```python
from build123d import *

# Parameters (mm, degrees)
F1_DEPTH = 20.6375
F2_W     = 9.525
F2_H     = 28.575
F3_DEPTH = 47.625
F4_W     = 9.525
F4_H     = 28.575
F5_DEPTH = 47.625
F6_W     = 1104.9
F6_H     = 7.9375
F7_DEPTH = 9.525


with BuildPart() as f1:
    # F0 (on Front) → F1 (new body)
    with BuildSketch(Plane.XZ):
        with BuildLine():
            Line((552.45, 0), (0, 0))
            Line((0, 0), (-552.45, 0))
            Line((-552.45, 0), (-552.45, -88.9))
            ThreePointArc((-552.45, -88.9), (0, -69.85), (552.45, -88.9))
            Line((552.45, -88.9), (552.45, 0))
        make_face()
    extrude(amount=-F1_DEPTH)

    # F2 (on face) → F3 (join)
    with BuildSketch(Plane(origin=(-552.45, 0, 0), x_dir=(0, -1, 0), z_dir=(-1, 0, 0))):
        with Locations((-10.31875, -23.8125)):
            Rectangle(F2_W, F2_H)
        with Locations((-10.31875, -65.0875)):
            Rectangle(F2_W, F2_H)
    extrude(amount=F3_DEPTH)

    # F4 (on face) → F5 (join)
    with BuildSketch(Plane.YZ.offset(552.45)):
        with Locations((10.31875, -23.8125)):
            Rectangle(F4_W, F4_H)
        with Locations((10.31875, -65.0875)):
            Rectangle(F4_W, F4_H)
    extrude(amount=F5_DEPTH)

    # F6 (on face) → F7 (cut)
    with BuildSketch(Plane.XY):
        with Locations((0, 10.31875)):
            Rectangle(F6_W, F6_H)
    extrude(amount=-F7_DEPTH, mode=Mode.SUBTRACT)


solid = f1.part
```
Here's how the part is built. I have some questions about the finished solid (model axes, mm). A direction names the side the tool comes from. Coordinates: 2 decimals unless noted, no trailing zeros. Order: outer loops, then holes, each group sorted by start corner. A loop starts at its lowest first (then second) coordinate and runs counter-clockwise, first axis right, second up. Notation, with made-up numbers: (36.5, 73.25) -> (61.5, 73.25) arc R31 cw to (61.5, 100.25) -> close; hole circle Ø5 at (61.25, 64.5). An arc over 180 degrees is marked (long way). Return JSON: item names as keys, results as strings.
1) I'm going to push flat-ended pins straight in: P1, Ø6, axis at y = 13.5, z = -46.5, coming from the +X side; P2, Ø5, axis at x = -576.5, y = 8, coming from the -Z side (3 decimals); P3, Ø23, axis at x = -587, z = -20.5, coming from the +Y side. Where does each tip first touch, or does it pass through?
Conclusion:
{"P1": "stops at x = 552.45", "P2": "stops at z = -79.375", "P3": "stops at y = 15.08"}
2) If we section it at A-A on y = 11: List the corners of the cut face in (x, z) for me (3 decimals), plus the area to 3 significant figures.
Conclusion:
{"outline": "(-600.075, -79.375) -> (-552.45, -79.375) -> (-552.45, -88.9) arc R8020.05 cw to (552.45, -88.9) -> (552.45, -79.375) -> (600.075, -79.375) -> (600.075, -50.8) -> (552.45, -50.8) -> (552.45, -38.1) -> (600.075, -38.1) -> (600.075, -9.525) -> (-600.075, -9.525) -> (-600.075, -38.1) -> (-552.45, -38.1) -> (-552.45, -50.8) -> (-600.075, -50.8) -> close", "area": "79,100 mm²"}
3) If I drill on probe 1 along X at (y, z) = (18.25, -30.5); probe 2 along Z at (x, y) = (-311.5, 5.75); probe 3 along Z at (x, y) = (-497, 8.5) (3 decimals), over which ranges is the centre line in solid material (lowest first)?
Conclusion:
{"probe 1": "x = -552.45 to 552.45", "probe 2": "z = -75.9 to 0", "probe 3": "z = -85.264 to -9.525"}
4) On a 3-axis mill with a long thin cutter (end or side, diameter ignored), from which of +Z, -Z, +X, -X, +Y, -Y can I reach the whole of each face in a straight line? I mean faces 1 (the flat face through (-576, 15.081, -65)), 2 (the flat face through (576, 15.081, -24)), 3 (the flat face through (576, 5.556, -65)). Say none if no direction works.
Conclusion:
{"face 1": "+Z, -Z, -X, +Y", "face 2": "+Z, -Z, +X, +Y", "face 3": "+Z, -Z, +X, -Y"}
5) Thinking about a two-plate mould opening in X: for faces 4 (the flat face through (576, 15.081, -65)), 5 (the cylindrical face through (-7.74, 10.174, -69.854)), which applies, +X half, -X half, draft (parallel to the pull), parting line (faces both ways), or undercut?
Conclusion:
{"face 4": "draft", "face 5": "undercut"}
